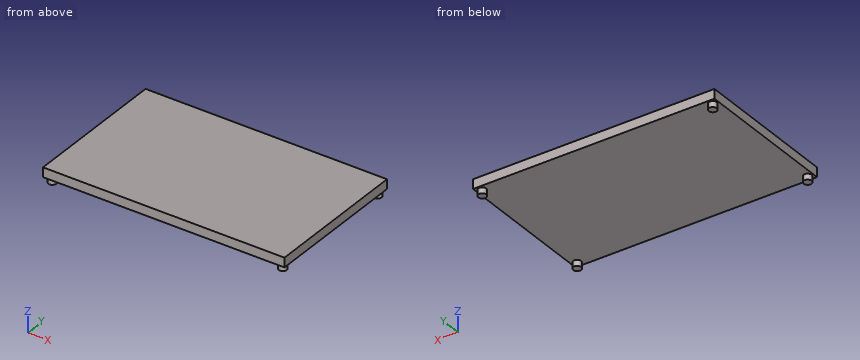
from build123d import *

# Parameters (mm, degrees)
SKETCH_1_W                                 = 165.5
SKETCH_1_H                                 = 100.5
EXTRUDE_1_DEPTH                            = 3.25
SKETCH_2_R                                 = 2.75
EXTRUDE_2_DEPTH                            = 4
MIRROR_1_AT_THE_SECOND_PLANE_COPY_1_SKET_R = 2.75
MIRROR_1_AT_THE_SECOND_PLANE_COPY_1_DEPTH  = 4


with BuildPart() as part:
    # 草图1 → 凸台-拉伸1 (new, symmetric)
    with BuildSketch(Plane.XY):
        Rectangle(SKETCH_1_W, SKETCH_1_H)
    extrude(amount=EXTRUDE_1_DEPTH, both=True)

    # 草图2 → 凸台-拉伸2 (add)
    with BuildSketch(Plane(origin=(0, 0, -3.25), x_dir=(-1, 0, 0), z_dir=(0, 0, -1))):
        with Locations((79, 46.5)):
            Circle(SKETCH_2_R)
    extrude_2 = extrude(amount=EXTRUDE_2_DEPTH)

    # 镜向1: 凸台-拉伸2 across plane
    add(extrude_2.mirror(Plane.ZX))

    # 镜向1 at the second plane: 凸台-拉伸2 across plane
    add(extrude_2.mirror(Plane(origin=(0, 0, 0), x_dir=(0, 0, 1), z_dir=(1, 0, 0))))

    # 镜向1 at the second plane copy 1 sket → 镜向1 at the second plane copy 1 (add)
    with BuildSketch(Plane(origin=(0, 0, -3.25), x_dir=(1, 0, 0), z_dir=(0, 0, -1))):
        with Locations((79, 46.5)):
            Circle(MIRROR_1_AT_THE_SECOND_PLANE_COPY_1_SKET_R)
    extrude(amount=MIRROR_1_AT_THE_SECOND_PLANE_COPY_1_DEPTH)


solid = part.part
Part model, mm, in its own coordinate system. Give positions to 0.01 mm unless a question says otherwise; leave off trailing zeros. Loops run counter-clockwise (first coordinate to the right, second up) from the corner with the lowest first, then second, coordinate; pieces in that order, holes last. Notation, with made-up numbers: (38.5, 7) -> (46.5, 7) arc R18 ccw to (46.5, 29) -> close; hole circle Ø11 at (71.25, 5.5). An arc over 180 degrees is marked (long way). Write each question's results on one line, items separated by ' | '. Start each with the question number.
Q1. Band-saw the part on C-C on x = 68.5. List the corners of the cut face in (y, z).
Q2. Band-saw the part on D-D on y = -17.5. List the corners of the cut face in (x, z).
Q3. Wall check: L1, parallel to Z at x = 53.5, y = -1.5; L2, parallel to X at y = -45.5, z = -5. Give the ranges that are in metal, low to high.
Q4. Band-saw the part on A-A on y = -46.5. List the corners of the cut face in (x, z), plus the area to 3 significant figures.
Q5. Band-saw the part on B-B on x = -79. List the corners of the cut face in (y, z), plus the area to 3 significant figures.
Q6. Pin check, flat tip, straight feed: P1, Ø12, axis at x = -37.5, y = -19, coming from the -Z side. Stop position of the tip, or through.
Results are:
1) outline: (-50.25, -3.25) -> (50.25, -3.25) -> (50.25, 3.25) -> (-50.25, 3.25) -> close
2) outline: (-82.75, -3.25) -> (82.75, -3.25) -> (82.75, 3.25) -> (-82.75, 3.25) -> close
3) L1: z = -3.25 to 3.25 | L2: x = -81.56 to -76.44, 76.44 to 81.56
4) outline: (-82.75, -3.25) -> (-81.75, -3.25) -> (-81.75, -7.25) -> (-76.25, -7.25) -> (-76.25, -3.25) -> (76.25, -3.25) -> (76.25, -7.25) -> (81.75, -7.25) -> (81.75, -3.25) -> (82.75, -3.25) -> (82.75, 3.25) -> (-82.75, 3.25) -> close | area: 1,120 mm²
5) outline: (-50.25, -3.25) -> (-49.25, -3.25) -> (-49.25, -7.25) -> (-43.75, -7.25) -> (-43.75, -3.25) -> (43.75, -3.25) -> (43.75, -7.25) -> (49.25, -7.25) -> (49.25, -3.25) -> (50.25, -3.25) -> (50.25, 3.25) -> (-50.25, 3.25) -> close | area: 697 mm²
6) P1: stops at z = -3.25
